Geometry: final body of the model. Coordinates: model frame, mm. Give positions to 0.01 mm unless a question says otherwise; leave off trailing zeros. Write each loop counter-clockwise with the first axis right and the second up, starting at its lowest first coordinate (ties: lowest second). Pieces come first, ordered by that corner, then holes. Notation, with made-up numbers: M 32.25,26.25 L 36.25,26.25 A21 cw 36.25,36.25 Z; hole C 36,6 d9. An arc over 180 degrees is marked long. Use a Markdown table: item, result. Add a question column.
(1) Cut plane A-A (y = 0). Output: boundary loops of the cut face in (x, z).
(2) Material intervals for L1, parallel to Z at x = 2.75, y = -0.5; L2, parallel to Z at x = 1.75, y = -1; L3, parallel to Y at x = 3, z = -152.4, sorted ascending.
(3) Pin query (flat end, axial travel): pin 1 Ø6 at (y, z) = (0, -85) entering from -X; pin 2 Ø2 at (x, y) = (2, -2) entering from -Z. Return the tip coordinate at first contact, or that it passes through.
```python
from build123d import *

# Parameters (mm, degrees)
SKETCH1_R           = 1.65
BOSS_EXTRUDE1_DEPTH = 6.35


with BuildPart() as part:
    # Sketch1 → Boss-Extrude1 (new body)
    with BuildSketch(Plane(origin=(0, 0, 0), x_dir=(0, 0, -1), z_dir=(1, 0, 0))):
        with BuildLine():
            Line((-152.4, 5), (152.4, 5))
            ThreePointArc((152.4, 5), (157.4, 0), (152.4, -5))
            Line((152.4, -5), (-152.4, -5))
            ThreePointArc((-152.4, -5), (-157.4, 0), (-152.4, 5))
        make_face()
        with Locations((-152.4, 0)):
            Circle(SKETCH1_R, mode=Mode.SUBTRACT)
        with Locations(Location((152.4, 0, 0), (0, 0, 180))):
            Circle(SKETCH1_R, mode=Mode.SUBTRACT)
    extrude(amount=BOSS_EXTRUDE1_DEPTH)


solid = part.part
```
Answer list:
| question | item | result |
|---|---|---|
| 1 | outline | M 0,-157.4 L 6.35,-157.4 L 6.35,-154.05 L 0,-154.05 Z; M 0,-150.75 L 6.35,-150.75 L 6.35,150.75 L 0,150.75 Z; M 0,154.05 L 6.35,154.05 L 6.35,157.4 L 0,157.4 Z |
| 2 | L1 | -157.37 to -153.97, -150.83 to 150.83, 153.97 to 157.37 |
| 2 | L2 | -157.3 to -153.71, -151.09 to 151.09, 153.71 to 157.3 |
| 2 | L3 | -5 to -1.65, 1.65 to 5 |
| 3 | pin 1 | x = 0 |
| 3 | pin 2 | z = -157.3 |
